Autodesk Inventor part; units mm, degrees
ref_plane "YZ Plane" through (0, 0, 0) normal (1, 0, 0) x (0, 1, 0)
ref_plane "XZ Plane" through (0, 0, 0) normal (0, 1, 0) x (-1, 0, 0)
ref_plane "XY Plane" through (0, 0, 0) normal (0, 0, 1) x (1, 0, 0)
sketch "Sketch1" plane through (0, 0, 0) normal (0, 1, 0) x (-1, 0, 0)
  circle A0 centre (0, 0) radius 10.414
  dimension "d0" = 20.828
extrude "Extrusion1" add sketch "Sketch1" along normal blind 2.286
sketch "Sketch2" plane through (0, 0, 0) normal (0, -1, 0) x (1, 0, 0)
  circle A0 centre (0, 0) radius 10.414
  circle A1 centre (0, 0) radius 4.064
  dimension "d3" = 8.128
extrude "Extrusion2" add sketch "Sketch2" along normal blind 4.064 contours A1
sketch "Sketch3" plane through (0, 2.286, 0) normal (0, 1, 0) x (1, 0, 0)
  circle A0 centre (0, 0) radius 10.414
  circle A1 centre (0, 0) radius 7.62 construction
  line L0 (-7.62, 0) -> (-7.62, -7.62) construction
  line L1 (-7.62, -7.62) -> (7.62, -7.62) construction
  line L2 (7.62, -7.62) -> (7.62, 7.62) construction
  line L3 (7.62, 7.62) -> (-7.62, 7.62) construction
  line L4 (-7.62, 7.62) -> (-7.62, 0) construction
  point P0 (0, 7.62)
  point P1 (3.81, 7.62)
  point P2 (-3.81, 7.62)
  point P3 (7.62, 0)
  point P4 (7.62, 3.81)
  point P5 (7.62, -3.81)
  point P6 (-7.62, 3.81)
  point P7 (-7.62, -3.81)
  point P8 (0, -7.62)
  point P9 (-3.81, -7.62)
  point P10 (3.81, -7.62)
  dimension "d6" = 15.24
  dimension "d8" = 7.62
  dimension "d9" = 7.62
  dimension "d10" = 7.62
  dimension "d11" = 3.81
  dimension "d12" = 3.81
  dimension "d13" = 3.81
  dimension "d14" = 3.81
  dimension "d15" = 3.81
  dimension "d16" = 3.81
  dimension "d17" = 3.81
  dimension "d18" = 3.81
hole "Hole1" at (0, 2.286, -7.62) at (3.81, 2.286, -7.62) at (-3.81, 2.286, -7.62) at (7.62, 2.286, 0) at (7.62, 2.286, -3.81) at (7.62, 2.286, 3.81) at (-7.62, 2.286, 0) at (-7.62, 2.286, -3.81) at (-7.62, 2.286, 3.81) at (0, 2.286, 7.62) at (-3.81, 2.286, 7.62) at (3.81, 2.286, 7.62) direction (0, -1, 0) diameter 1.4732 end through all
hole "Hole2" at (0, 2.286, 0) direction (0, -1, 0) diameter 3.048 end through all
properties part number "horn01" material "Aluminum 6061"
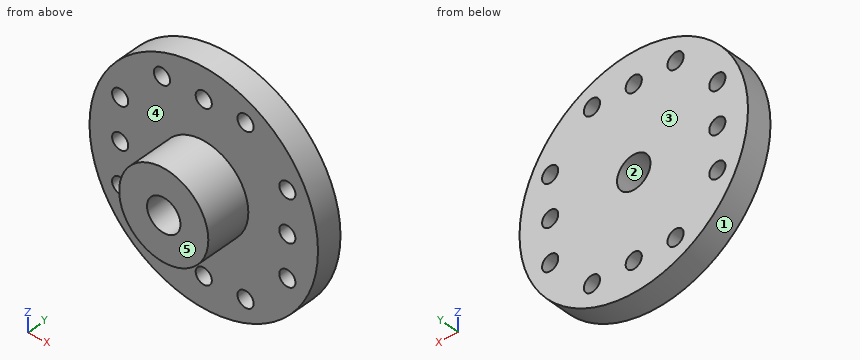
CAD build for the part. Positions are in the model's coordinates, mm. Face numbers are marked on the shaded views. A direction names the side the tool comes from. Coordinates: 2 decimals unless noted, no trailing zeros. Write each loop counter-clockwise with the first axis right and the second up, starting at its lowest first coordinate (ties: lowest second). Pieces come first, ordered by that corner, then holes. Notation, with made-up numbers: M 21,32 L 61,32 A20 ccw 61,47 Z; hole C 13,32 d6. An arc over 180 degrees is marked long. Answer as a JSON object with one key per item and string values. Group by question number.
1) Tool access for the marked faces 4 and 5: list every direction of +Z, -Z, +X, -X, +Y, -Y with a clear straight run to the whole face (end or side of a thin tool).
2) Pin check, flat tips, straight feed: pin 1 Ø1.7 at (x, z) = (-7.62, -3.81) entering from +Y; pin 2 Ø1.2 at (x, z) = (7.62, 0) entering from -Y; pin 3 Ø2 at (x, y) = (2, 1.5) entering from +Z; pin 4 Ø2.5 at (x, z) = (0, 7.62) entering from -Y. Stop position of each tip, or through.
3) Saw through at C-C (y = 0.25). Give the number of separate pieces and of enclosed holes in the cut face, plus the area to 3 significant figures.
4) Wall check: line 1 (X direction, y = 1.7, z = -3.81); line 2 (X direction, y = 1.5, z = -7.25); line 3 (Z direction, x = 7.62, y = 1.4). Give the ranges that are in metal, low to high. Write a range as from..to.
5) Saw through at B-B (z = 0). Write the cut outline in (x, y), plus the area to 3 significant figures.
6) Saw through at D-D (x = -3.81). Write the cut outline in (y, z), plus the area to 3 significant figures.
7) Mould opens along Z. For the marked faces 1, 2 and 3 say: +Z half, -Z half, draft (parallel to the pull), parting line (faces both ways), or undercut.
8) Saw through at A-A (x = 0). Write the cut outline in (y, z), plus the area to 3 significant figures.
Values follow:
{
 "1": {"face 4": "-Y", "face 5": "+Z, -Z, +X, -X, -Y"},
 "2": {"pin 1": "stops at y = 2.29", "pin 2": "passes through", "pin 3": "stops at z = 10.37", "pin 4": "stops at y = 0"},
 "3": {"separate pieces": "1", "enclosed holes": "13", "area": "313 mm2"},
 "4": {"line 1": "x = -9.69..-8.36, -6.88..6.88, 8.36..9.69", "line 2": "x = -7.48..-4.45, -3.17..-0.64, 0.64..3.17, 4.45..7.48", "line 3": "z = -7.1..-4.55, -3.07..-0.74, 0.74..3.07, 4.55..7.1"},
 "5": {"outline": "M -10.41,0 L -8.36,0 L -8.36,2.29 L -10.41,2.29 Z; M -6.88,0 L -4.06,0 L -4.06,-4.06 L -1.52,-4.06 L -1.52,2.29 L -6.88,2.29 Z; M 1.52,-4.06 L 4.06,-4.06 L 4.06,0 L 6.88,0 L 6.88,2.29 L 1.52,2.29 Z; M 8.36,0 L 10.41,0 L 10.41,2.29 L 8.36,2.29 Z", "area": "54.6 mm2"},
 "6": {"outline": "M -4.06,-1.41 L 0,-1.41 L 0,-6.88 L 2.29,-6.88 L 2.29,6.88 L 0,6.88 L 0,1.41 L -4.06,1.41 Z; M 0,-9.69 L 2.29,-9.69 L 2.29,-8.36 L 0,-8.36 Z; M 0,8.36 L 2.29,8.36 L 2.29,9.69 L 0,9.69 Z", "area": "49.1 mm2"},
 "7": {"face 1": "parting line", "face 2": "undercut", "face 3": "draft"},
 "8": {"outline": "M -4.06,-4.06 L 0,-4.06 L 0,-6.88 L 2.29,-6.88 L 2.29,-1.52 L -4.06,-1.52 Z; M -4.06,1.52 L 2.29,1.52 L 2.29,6.88 L 0,6.88 L 0,4.06 L -4.06,4.06 Z; M 0,-10.41 L 2.29,-10.41 L 2.29,-8.36 L 0,-8.36 Z; M 0,8.36 L 2.29,8.36 L 2.29,10.41 L 0,10.41 Z", "area": "54.6 mm2"}
}
